Source: CAD feature listing. Evaluate the final solid. Frame: model axes, mm. A direction names the side the tool comes from. Coordinates: 2 decimals unless noted, no trailing zeros. Loops run counter-clockwise (first coordinate to the right, second up) from the corner with the lowest first, then second, coordinate; pieces in that order, holes last. Notation, with made-up numbers: (20, -7) -> (38, -7) arc R13 ccw to (38, 9) -> close; hole circle Ø4 at (15.25, 28.5). An arc over 180 degrees is marked (long way). Answer as a JSON object with one key per item and string values. Group by question number.
from build123d import *

# Parameters (mm, degrees)
BOSS_EXTRUDE1_DEPTH = 5.08
FILLET1_R           = 2.54
SKETCH5_R           = 0.889
SKETCH5_W           = 12.7
SKETCH5_H           = 23.114
CUT_EXTRUDE1_DEPTH  = 35.323380204


with BuildPart() as part:
    # Sketch1 → Boss-Extrude1 (new body)
    with BuildSketch(Plane.XY):
        with BuildLine():
            Line((-6.985, 11.9888), (6.985, 11.9888))
            ThreePointArc((6.985, 11.9888), (16.273931797, 9.848966937), (23.69046712, 3.8608))
            ThreePointArc((23.69046712, 3.8608), (0, -24.003), (-23.69046712, 3.8608))
            ThreePointArc((-23.69046712, 3.8608), (-16.273931797, 9.848966937), (-6.985, 11.9888))
        make_face()
    extrude(amount=BOSS_EXTRUDE1_DEPTH)

    # Fillet1
    fillet1_edges = [part.edges().sort_by_distance(p)[0] for p in [
        (23.69046712, 3.8608, 2.54),
        (-23.69046712, 3.8608, 2.54),
    ]]
    fillet(fillet1_edges, radius=FILLET1_R)

    # Sketch5 → Cut-Extrude1 (cut, through all)
    with BuildSketch(Plane.XY.offset(5.08)):
        with Locations((0, -16.54175)):
            Circle(SKETCH5_R)
        with Locations((0, 11.05535)):
            Circle(SKETCH5_R)
        with Locations((0, -2.7432)):
            Rectangle(SKETCH5_W, SKETCH5_H)
    extrude(amount=-CUT_EXTRUDE1_DEPTH, mode=Mode.SUBTRACT)


solid = part.part
1. Section query A-A on x = 0. Return loops of the section in (y, z).
2. Section query D-D on z = 4.4. State how many separate pieces and enclosed holes the cut face has, then the cut area to 3 significant figures.
3. Pin query (flat end, axial travel): pin 1 Ø2 at (x, z) = (12, 2.5) entering from -Y; pin 2 Ø2 at (y, z) = (4, 4) entering from +X; pin 3 Ø3 at (y, z) = (7.5, 4) entering from -X. Return the tip coordinate at first contact, or that it passes through.
4. Ray query, L1, parallel to X at y = -5.5, z = 3.8; L2, parallel to X at y = 8, z = 3.35; L3, parallel to Y at x = 12.5, z = 1.5. Return the intervals inside material, ascending.
5. Section query C-C on x = -5. Return loops of the section in (y, z).
6. Section query B-B on y = -4. Return loops of the section in (x, z).
7. Reachability of faces 4 (the face through (0, -14.3, 3)), 5 (the face through (-10, -6, 5.08)) from +Z, -Z, +X, -X, +Y, -Y: full face, straight path, thin tool, end or side. Return the list, or none.
8. Mould query, pull axis Y, two halves, no side actions, for faces 1 (the face through (-10, -6, 0)), 2 (the face through (-2, 11.989, 3)), 3 (the face through (0, 8.814, 3)). Classes: pulls with the +Y half, pulls with the -Y half, needs draft (parallel to the pull), parting line crosses it, or undercut.
Solved:
{
 "1": {"outline": "(-24, 0) -> (-17.43, 0) -> (-17.43, 5.08) -> (-24, 5.08) -> close; (-15.65, 0) -> (-14.3, 0) -> (-14.3, 5.08) -> (-15.65, 5.08) -> close; (8.81, 0) -> (10.17, 0) -> (10.17, 5.08) -> (8.81, 5.08) -> close; (11.94, 0) -> (11.99, 0) -> (11.99, 5.08) -> (11.94, 5.08) -> close"},
 "2": {"separate pieces": "1", "enclosed holes": "3", "area": "1,090 mm^2"},
 "3": {"pin 1": "y = -21.33", "pin 2": "x = 23.81", "pin 3": "x = -21.76"},
 "4": {"L1": "-23.36 to -6.35, 6.35 to 23.36", "L2": "-19.37 to -6.35, 6.35 to 19.37", "L3": "-20.49 to 11.26"},
 "5": {"outline": "(-23.48, 0) -> (-14.3, 0) -> (-14.3, 5.08) -> (-23.48, 5.08) -> close; (8.81, 0) -> (11.99, 0) -> (11.99, 5.08) -> (8.81, 5.08) -> close"},
 "6": {"outline": "(-23.67, 0) -> (-6.35, 0) -> (-6.35, 5.08) -> (-23.67, 5.08) -> close; (6.35, 0) -> (23.67, 0) -> (23.67, 5.08) -> (6.35, 5.08) -> close"},
 "7": {"face 4": "+Z, -Z", "face 5": "+Z, +X, -X, +Y, -Y"},
 "8": {"face 1": "needs draft", "face 2": "pulls with the +Y half", "face 3": "undercut"}
}
